Read the model definition and answer for the solid it produces. Units are mm, in the model's axes. Face numbers are marked on the shaded views. A direction names the side the tool comes from. Give positions to 0.01 mm unless a question says otherwise; leave off trailing zeros. Order: outer loops, then holes, each group sorted by start corner. A loop starts at its lowest first (then second) coordinate and runs counter-clockwise, first axis right, second up. Notation, with made-up numbers: (-12.75, 82) - (39.25, 82) arc R34 cw to (39.25, 116) - close; hole circle Ø7 at (-14, 89.25). An arc over 180 degrees is marked (long way). Return JSON: item names as keys, results as strings.
Autodesk Inventor part; units mm, degrees
ref_plane "YZ Plane" through (0, 0, 0) normal (1, 0, 0) x (0, 1, 0)
ref_plane "XZ Plane" through (0, 0, 0) normal (0, 1, 0) x (-1, 0, 0)
ref_plane "XY Plane" through (0, 0, 0) normal (0, 0, 1) x (1, 0, 0)
sketch "スケッチ1" plane through (0, 0, 0) normal (0, 0, 1) x (1, 0, 0)
  circle A0 centre (45.6488, -28.0072) radius 8
  circle A1 centre (45.6488, -28.0072) radius 7 construction
  line L0 (45.6488, -21.0072) -> (51.7109, -24.5072) construction
  line L1 (51.7109, -24.5072) -> (51.7109, -31.5072) construction
  line L2 (51.7109, -31.5072) -> (45.6488, -35.0072) construction
  line L3 (45.6488, -35.0072) -> (39.5866, -31.5072) construction
  line L4 (39.5866, -31.5072) -> (39.5866, -24.5072) construction
  line L5 (39.5866, -24.5072) -> (45.6488, -21.0072) construction
  arc A2 (47.3808, -22.0072) -> (43.9167, -22.0072) centre (45.6488, -23.0072) ccw
  arc A3 (41.3186, -23.5072) -> (39.5866, -26.5072) centre (41.3186, -25.5072) ccw
  arc A4 (39.5866, -29.5072) -> (41.3186, -32.5072) centre (41.3186, -30.5072) ccw
  arc A5 (43.9167, -34.0072) -> (47.3808, -34.0072) centre (45.6488, -33.0072) ccw
  arc A6 (49.9789, -32.5072) -> (51.7109, -29.5072) centre (49.9789, -30.5072) ccw
  arc A7 (51.7109, -26.5072) -> (49.9789, -23.5072) centre (49.9789, -25.5072) ccw
  arc A8 (47.3808, -22.0072) -> (49.9789, -23.5072) centre (49.9789, -20.5072) ccw
  arc A9 (41.3186, -23.5072) -> (43.9167, -22.0072) centre (41.3186, -20.5072) ccw
  arc A10 (39.5866, -29.5072) -> (39.5866, -26.5072) centre (36.9885, -28.0072) ccw
  arc A11 (43.9167, -34.0072) -> (41.3186, -32.5072) centre (41.3186, -35.5072) ccw
  arc A12 (49.9789, -32.5072) -> (47.3808, -34.0072) centre (49.9789, -35.5072) ccw
  arc A13 (51.7109, -26.5072) -> (51.7109, -29.5072) centre (54.309, -28.0072) ccw
  circle A14 centre (45.6488, -28.0072) radius 5.6603 construction
  point P0 (0, 0)
  point P1 (51.7109, -31.5072)
  point P2 (51.7109, -24.5072)
  point P3 (39.5866, -26.5072)
  point P4 (41.3186, -23.5072)
  point P5 (43.9167, -22.0072)
  point P6 (51.7109, -26.5072)
  dimension "d5" = 14
  dimension "d4" = 16
  dimension "d6" = 360
  dimension "d7" = 360
  dimension "d8" = 11.3205
  dimension "d9" = 3
  dimension "d10" = 2
extrude "押し出し1" add sketch "スケッチ1" along normal blind 5
properties part number "1ギア接続部外" material "アルミニウム 2014-T4"
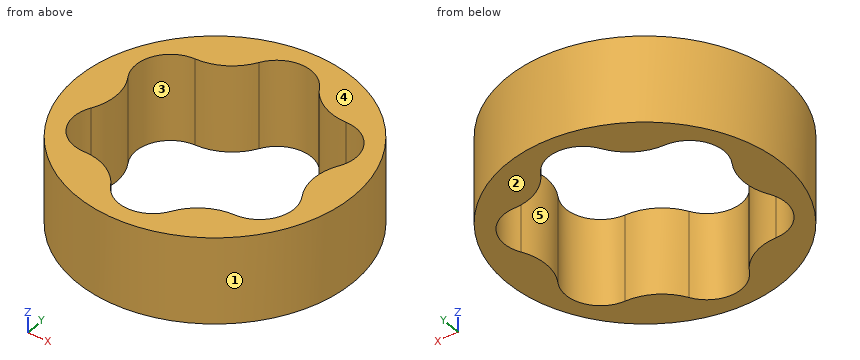
Q1. A cutting plane is placed at A-A (y = -31.5). Write down the section's boundary in (x, z).
Values:
{"outline": "(38.45, 0) - (39.58, 0) - (39.58, 5) - (38.45, 5) - close; (51.72, 0) - (52.85, 0) - (52.85, 5) - (51.72, 5) - close"}
Q2. Given pin 1 (2 mm diameter, centred on y = -26.5, z = 1.5, fed in from +X); pin 2 (2 mm diameter, centred on x = 51.5, z = 3.5, fed in from +Y), each flat-ended and moving along its own axis, determine where each tip first touches the part or whether it passes through.
Values:
{"pin 1": "stops at x = 53.63", "pin 2": "stops at y = -21.65"}
Q3. For the marked faces 4 and 5, determine the directions among +Z, -Z, +X, -X, +Y, -Y from which every point of the face is accessible in a straight line to the end or side of a thin tool.
Values:
{"face 4": "+Z, +X, -X, +Y, -Y", "face 5": "+Z, -Z"}
Q4. Determine the mould class of the marked faces 1, 2 and 3 for opening direction Y: released by +Y, released by -Y, zero draft, split by the parting line, or undercut.
Values:
{"face 1": "split by the parting line", "face 2": "zero draft", "face 3": "undercut"}
Q5. A cutting plane is placed at D-D (x = 38.75). Write down the section's boundary in (y, z), and give its area (3 significant figures).
Values:
{"outline": "(-32.06, 0) - (-23.96, 0) - (-23.96, 5) - (-32.06, 5) - close", "area": "40.5 mm²"}
Q6. A cutting plane is placed at C-C (z = 4.25). Write down the section's boundary in (x, y), and give its area (3 significant figures).
Values:
{"outline": "circle Ø16 at (45.65, -28.01); hole (39.59, -29.51) arc R2 ccw to (41.32, -32.51) arc R3 cw to (43.92, -34.01) arc R2 ccw to (47.38, -34.01) arc R3 cw to (49.98, -32.51) arc R2 ccw to (51.71, -29.51) arc R3 cw to (51.71, -26.51) arc R2 ccw to (49.98, -23.51) arc R3 cw to (47.38, -22.01) arc R2 ccw to (43.92, -22.01) arc R3 cw to (41.32, -23.51) arc R2 ccw to (39.59, -26.51) arc R3 cw to start", "area": "74.3 mm²"}
Q7. Consider L1, parallel to X at y = -25, z = 0.85; L2, parallel to X at y = -26.25, z = 1.5; L3, parallel to Y at x = 40.75, z = 3.65. Determine where each line is inside the solid, lowest interval first.
Values:
{"L1": "x = 38.24 to 39.38, 51.91 to 53.06", "L2": "x = 37.84 to 39.46, 51.84 to 53.45", "L3": "y = -34.33 to -32.42, -23.59 to -21.68"}
Q8. A cutting plane is placed at B-B (x = 46.75). Write down the section's boundary in (y, z).
Values:
{"outline": "(-35.93, 0) - (-34.68, 0) - (-34.68, 5) - (-35.93, 5) - close; (-21.34, 0) - (-20.08, 0) - (-20.08, 5) - (-21.34, 5) - close"}
